```python
from build123d import *

# Parameters (mm, degrees)
F0_W     = 38
F0_H     = 38
F1_DEPTH = 2.5
F3_DEPTH = 9
F4_SIZE2 = 5
F4_SIZE  = 1
F6_COUNT = 4
F7_R     = 1


with BuildPart() as f1:
    # F0 (on Top) → F1 (new body)
    with BuildSketch(Plane.XY):
        Rectangle(F0_W, F0_H)
    extrude(amount=F1_DEPTH)



with BuildPart() as f3:
    # F2 (on face) → F3 (new body)
    with BuildSketch(Plane.XY.offset(2.5)):
        Polygon((-15.5, 0), (-13.5, 0), (-13.5, 8.5), (-8.5, 8.5), (-8.5, 13.5), (0, 13.5), (0, 15.5), (-2.5, 15.5), (-2.5, 17.5), (-6.5, 17.5), (-6.5, 15.5), (-10.5, 15.5), (-10.5, 10.5), (-15.5, 10.5), (-15.5, 6.5), (-17.5, 6.5), (-17.5, 2.5), (-15.5, 2.5), align=None)
    extrude(amount=F3_DEPTH)

    # F4
    f4_edges = [f3.edges().sort_by_distance(p)[0] for p in [
        (-17.5, 4.5, 11.5),
        (-4.5, 17.5, 11.5),
    ]]
    f4_side = f3.faces().sort_by_distance((-10.131757, 10.131757, 11.5))[0]
    chamfer(f4_edges, length=F4_SIZE, length2=F4_SIZE2, reference=f4_side)


with BuildPart() as f1_1:
    add(f1.part)

    add(f3.part)  # F6 merges F3
    # F6: F3 ×4 about axis
    f6_axis = Axis((0, 0, 21.3143786676), (0, 0, 1))
    for i in range(1, F6_COUNT):
        add(f3.part.rotate(f6_axis, i * 360 / F6_COUNT))

    # F7
    f7_edges = [f1_1.edges().sort_by_distance(p)[0] for p in [
        (0, 19, 0),
        (-19, 0, 0),
        (0, -19, 0),
        (19, 0, 0),
    ]]
    fillet(f7_edges, radius=F7_R)


solid = f1_1.part
```
Geometry check sheet. Reference: the model listing, model coordinates, mm. A direction names the side the tool comes from. Coordinates: 2 decimals unless noted, no trailing zeros. Order: outer loops, then holes, each group sorted by start corner. A loop starts at its lowest first (then second) coordinate and runs counter-clockwise, first axis right, second up. Notation, with made-up numbers: (13, 49) - (28, 49) arc R23 cw to (28, 70) - close; hole circle Ø10 at (84, -10.75). An arc over 180 degrees is marked (long way). Answer in a Markdown table with one row per item. Add a question column.
1. Section check C-C (y = -11). Enter the section's corners in (x, z).
2. Access from +Z, -Z, +X, -X, +Y, -Y to the whole of each face (thin tool, end or side, straight path). Record for faces 1 (the face through (-17.5, 5, 4)), 2 (the face through (-10.5, -13, 7)), 3 (the face through (-16, -2.5, 7)), 4 (the face through (-11, -8.5, 7)), 5 (the face through (13, 10.5, 7)).
3. Draft check along X on faces 6 (the face through (-16, 6.5, 7)), 7 (the face through (-15.5, -8, 7)), 8 (the face through (11, -8.5, 7)). Enter one of: +X half, -X half, draft (parallel to the pull), parting line (faces both ways), or undercut.
4. Material ranges on L1, parallel to Y at x = -16, z = 8; L2, parallel to X at y = 12, z = 10; L3, parallel to Y at x = 9.5, z = 3, recorded low to high. Write a range as [from, to].
5. Section check A-A (y = -17). Enter the section's corners in (x, z), plus the area to 3 significant figures.
6. Section check B-B (x = -4). Enter the section's corners in (y, z), plus the area to 3 significant figures.
7. Gauge pin test, flat ends, axial feed: pin 1 Ø5 at (y, z) = (2.5, 9.5) entering from +X; pin 2 Ø2.5 at (y, z) = (13.5, 6) entering from -X; pin 3 Ø1 at (y, z) = (-10.5, 8) entering from -X. Record the tip position at first contact, or that the pin passes through.
Data:
| question | item | result |
|---|---|---|
| 1 | outline | (-19, 1) arc R1 ccw to (-18, 0) - (18, 0) arc R1 ccw to (19, 1) - (19, 2.5) - (10.5, 2.5) - (10.5, 11.5) - (8.5, 11.5) - (8.5, 2.5) - (-8.5, 2.5) - (-8.5, 11.5) - (-10.5, 11.5) - (-10.5, 2.5) - (-19, 2.5) - close |
| 2 | face 1 | +Z, -X, +Y, -Y |
| 2 | face 2 | +Z, -X, -Y |
| 2 | face 3 | +Z, -X |
| 2 | face 4 | +Z |
| 2 | face 5 | +Z, +X, +Y |
| 3 | face 6 | draft |
| 3 | face 7 | -X half |
| 3 | face 8 | undercut |
| 4 | L1 | y = [-6.5, -2.5], [2.5, 6.5] |
| 4 | L2 | x = [-10.5, -8.5], [8.5, 10.5] |
| 4 | L3 | y = [-15.5, -8.5], [8.5, 15.5] |
| 5 | outline | (-19, 1) arc R1 ccw to (-18, 0) - (18, 0) arc R1 ccw to (19, 1) - (19, 2.5) - (6.5, 2.5) - (6.5, 9) - (2.5, 9) - (2.5, 2.5) - (-2.5, 2.5) - (-2.5, 9) - (-6.5, 9) - (-6.5, 2.5) - (-19, 2.5) - close |
| 5 | area | 147 mm² |
| 6 | outline | (-19, 1) arc R1 ccw to (-18, 0) - (18, 0) arc R1 ccw to (19, 1) - (19, 2.5) - (17.5, 2.5) - (17.5, 6.5) - (16.5, 11.5) - (13.5, 11.5) - (13.5, 2.5) - (-13.5, 2.5) - (-13.5, 11.5) - (-16.5, 11.5) - (-17.5, 6.5) - (-17.5, 2.5) - (-19, 2.5) - close |
| 6 | area | 162 mm² |
| 7 | pin 1 | stops at x = 17.4 |
| 7 | pin 2 | stops at x = -10.5 |
| 7 | pin 3 | stops at x = -15.5 |
